```python
from build123d import *

# Parameters (mm, degrees)
SKETCH_1_R          = 20
SKETCH_1_R_2        = 10
EXTRUDE_1_DEPTH     = 14
SKETCH_2_W          = 12
SKETCH_2_H          = 2
CUT_EXTRUDE_1_DEPTH = 32.559467676
SKETCH_4_R          = 2.25
CUT_EXTRUDE_3_DEPTH = 14


with BuildPart() as part:
    # 草图1 → 凸台-拉伸1 (new body)
    with BuildSketch(Plane.XY.offset(-7)):
        Circle(SKETCH_1_R)
        Circle(SKETCH_1_R_2, mode=Mode.SUBTRACT)
    extrude(amount=EXTRUDE_1_DEPTH)

    # 草图2 → 切除-拉伸1 (cut, through all)
    with BuildSketch(Plane.XY.offset(-7)):
        with Locations((15, 0)):
            Rectangle(SKETCH_2_W, SKETCH_2_H)
    extrude(amount=CUT_EXTRUDE_1_DEPTH, mode=Mode.SUBTRACT)

    # 草图4 → 切除-拉伸3 (cut)
    with BuildSketch(Plane(origin=(0, -7, 0), x_dir=(1, 0, 0), z_dir=(0, 1, 0))):
        with Locations(Location((15, 0, 0), (0, 0, 270))):
            Circle(SKETCH_4_R)
    extrude(amount=CUT_EXTRUDE_3_DEPTH, mode=Mode.SUBTRACT)


solid = part.part
```
Model file for the job. Use its own axes, mm. A direction names the side the tool comes from. Coordinates: 2 decimals unless noted, no trailing zeros. Write each loop counter-clockwise with the first axis right and the second up, starting at its lowest first coordinate (ties: lowest second). Pieces come first, ordered by that corner, then holes. Notation, with made-up numbers: (55, -19.5) - (75, -19.5) arc R10 cw to (75, -14.5) - close; hole circle Ø2 at (-39.75, 18). An arc over 180 degrees is marked (long way). Use a Markdown table: item, result. Add a question column.
Item 1: Drill centre lines: line 1 along Y through (x, z) = (0, -2.75); line 2 along X through (y, z) = (2.3, 0); line 3 along X through (y, z) = (2.9, 0). Where is each one in solid material? Low to high.
Item 2: Band-saw the part on D-D, the plane z = 0. Write the cut outline in (x, y).
Item 3: Drop flat-ended pins along their axis: pin 1 (2 mm diameter, centred on x = 16, z = 5.5, fed in from +Y); pin 2 (5 mm diameter, centred on x = 15, z = -3, fed in from -Y); pin 3 (5 mm diameter, centred on y = -6.5, z = -2, fed in from +X); pin 4 (4 mm diameter, centred on x = -6, y = -1, fed in from +Z). Give the stop position or say it passes through.
Item 4: Band-saw the part on B-B, the plane y = 2. Write the cut outline in (x, z).
Item 5: Band-saw the part on C-C, the plane y = 7.5. Write the cut outline in (x, z), and give its area (3 significant figures).
Item 6: 3-axis set-ups, long thin cutter, end or side, ignore diameter. For faces 1 (the face through (15, 7, 0)), 2 (the face through (-10, 0, 0)), 3 (the face through (13, -1, -2)): which of +Z, -Z, +X, -X, +Y, -Y reach the whole face in a straight line?
Item 7: Two-plate mould, pull along X, no slides. Class faces 4 (the face through (-19.98, 0.87, -0.1)), 5 (the face through (12.804, 3.958, -0.488)), 6 (the face through (13, 1, -2)): pulls with the +X half, pulls with the -X half, needs draft (parallel to the pull), parting line crosses it, or undercut.
Item 8: Band-saw the part on A-A, the plane x = 0. Write the cut outline in (y, z), and give its area (3 significant figures).
A:
| question | item | result |
|---|---|---|
| 1 | line 1 | y = -20 to -10, 10 to 20 |
| 1 | line 2 | x = -19.87 to -9.73, 9.73 to 12.75, 17.25 to 19.87 |
| 1 | line 3 | x = -19.79 to -9.57, 9.57 to 12.75, 17.25 to 19.79 |
| 2 | outline | (9.95, -1) arc R10 cw (long way) to (9.95, 1) - (12.75, 1) - (12.75, 7) - (17.25, 7) - (17.25, 1) - (19.97, 1) arc R20 ccw (long way) to (19.97, -1) - (17.25, -1) - (17.25, -7) - (12.75, -7) - (12.75, -1) - close |
| 3 | pin 1 | stops at y = 13.23 |
| 3 | pin 2 | stops at y = -15.61 |
| 3 | pin 3 | stops at x = 19.6 |
| 3 | pin 4 | passes through |
| 4 | outline | (-19.9, -7) - (-9.8, -7) - (-9.8, 7) - (-19.9, 7) - close; (9.8, -7) - (19.9, -7) - (19.9, 7) - (9.8, 7) - close; hole circle Ø4.5 at (15, 0) |
| 5 | outline | (-18.54, -7) - (-6.61, -7) - (-6.61, 7) - (-18.54, 7) - close; (6.61, -7) - (18.54, -7) - (18.54, 7) - (6.61, 7) - close |
| 5 | area | 334 mm² |
| 6 | face 1 | none |
| 6 | face 2 | +Z, -Z |
| 6 | face 3 | +Z, -Z, +X |
| 7 | face 4 | parting line crosses it |
| 7 | face 5 | undercut |
| 7 | face 6 | needs draft |
| 8 | outline | (-20, -7) - (-10, -7) - (-10, 7) - (-20, 7) - close; (10, -7) - (20, -7) - (20, 7) - (10, 7) - close |
| 8 | area | 280 mm² |
